```python
from build123d import *

# Parameters (mm, degrees)
BOSS_EXTRUDE1_DEPTH       = 15.875
SHELL1_T                  = -8.89
SKETCH2_R                 = 3.175
CUT_EXTRUDE1_DEPTH        = 7.35
F_4_40_TAPPED_HOLE1_D     = 2.2606
F_4_40_TAPPED_HOLE1_DEPTH = 7.62
F_4_40_TAPPED_HOLE1_TIP   = 0.679153


with BuildPart() as part:
    # Sketch1 → Boss-Extrude1 (new body, symmetric)
    with BuildSketch(Plane.XY):
        with BuildLine():
            ThreePointArc((0, -50.8), (-35.921024, -35.921024), (-50.8, 0))
            Line((-50.8, 0), (-67.31, 0))
            Line((-67.31, 0), (-67.31, -118.11))
            Line((-67.31, -118.11), (-88.9, -118.11))
            Line((-88.9, -118.11), (-88.9, -124.46))
            Line((-88.9, -124.46), (0, -124.46))
            Line((0, -124.46), (0, -50.8))
        make_face()
        with BuildLine():
            ThreePointArc((50.8, 0), (35.921024, -35.921024), (0, -50.8))
            Line((0, -50.8), (0, -124.46))
            Line((0, -124.46), (88.9, -124.46))
            Line((88.9, -124.46), (88.9, -118.11))
            Line((88.9, -118.11), (67.31, -118.11))
            Line((67.31, -118.11), (67.31, 0))
            Line((67.31, 0), (50.8, 0))
        make_face()
    extrude(amount=BOSS_EXTRUDE1_DEPTH, both=True)

    # Shell1
    shell1_openings = [part.faces().sort_by_distance(p)[0] for p in [
        (0, -77.216, 15.875),
        (0, -77.216, -15.875),
    ]]
    offset(amount=SHELL1_T, openings=shell1_openings)

    # Sketch2 → Cut-Extrude1 (cut, through all)
    with BuildSketch(Plane(origin=(0, -118.11, 0), x_dir=(1, 0, 0), z_dir=(0, 1, 0))):
        with Locations((-78.105, 0)):
            Circle(SKETCH2_R)
        with Locations((78.105, 0)):
            Circle(SKETCH2_R)
    extrude(amount=-CUT_EXTRUDE1_DEPTH, mode=Mode.SUBTRACT)

    # #4-40 Tapped Hole1
    with Locations(Plane(origin=(0, 0, 0), x_dir=(1, 0, 0), z_dir=(0, 1, 0))):
        with Locations((-57.658, 5.715), (-57.658, -6.985), (57.658, -6.985), (57.658, 5.715)):
            Hole(F_4_40_TAPPED_HOLE1_D / 2, depth=F_4_40_TAPPED_HOLE1_DEPTH)
            with Locations((0, 0, -(F_4_40_TAPPED_HOLE1_DEPTH + F_4_40_TAPPED_HOLE1_TIP / 2))):  # 118° drill point
                Cone(0, F_4_40_TAPPED_HOLE1_D / 2, F_4_40_TAPPED_HOLE1_TIP, mode=Mode.SUBTRACT)


solid = part.part
```
Read the model definition and answer for the solid it produces. Units are mm, in the model's axes. A direction names the side the tool comes from. Round coordinates to 2 decimals unless told otherwise and drop trailing zeros. Write each loop counter-clockwise with the first axis right and the second up, starting at its lowest first coordinate (ties: lowest second). Pieces come first, ordered by that corner, then holes. Notation, with made-up numbers: (48, 10) - (53, 10) arc R20 ccw to (53, 25) - close; hole circle Ø7 at (37, 4). An arc over 180 degrees is marked (long way). Use CSV: the item, a comma, the result in double quotes.
Q1. A tool of negligible diameter and unlimited length cuts with its end or side. For faces 4 (the flat face through (-58.42, -63, 0)), 5 (the flat face through (67.31, -60, 0)), 6 (the flat face through (-67.31, -58, 0)), from which of +Z, -Z, +X, -X, +Y, -Y can it reach the whole face along a straight path? Write none if from no direction.
Values:
face 4,"+Z, -Z"
face 5,"+Z, -Z, +X, +Y"
face 6,"+Z, -Z, -X, +Y"
Q2. Find section B-B, the plane y = -62.5. Write down the section's boundary in (x, z) (3 decimals), then the cut area to 3 significant figures.
Values:
outline,"(-67.31, -15.875) - (-58.42, -15.875) - (-58.42, 15.875) - (-67.31, 15.875) - close; (58.42, -15.875) - (67.31, -15.875) - (67.31, 15.875) - (58.42, 15.875) - close"
area,"565 mm²"
Q3. Determine the mould class of faces 1 (the cylindrical face through (-81.277, -121.241, -0.14)), 2 (the flat face through (58.42, -65, 0)), 3 (the flat face through (78, -118.11, 4)) for opening direction Y: +Y half, -Y half, draft (parallel to the pull), parting line (faces both ways), or undercut.
Values:
face 1,"draft"
face 2,"undercut"
face 3,"+Y half"
Q4. Straight lines are drawn through the part: line 1 along X through (y, z) = (-122, 0); line 2 along X through (y, z) = (-86.5, -12.5); line 3 along X through (y, z) = (-119, -2.5). For each, find the intervals that lie inside material, in ascending order.
Values:
line 1,"x = -88.9 to -81.28, -74.93 to 74.93, 81.28 to 88.9"
line 2,"x = -67.31 to -58.42, 58.42 to 67.31"
line 3,"x = -88.9 to -80.06, -76.15 to 76.15, 80.06 to 88.9"
Q5. Find section A-A, the plane z = 0. Write down the section's boundary in (x, y), then the cut area to 3 significant figures.
Values:
outline,"(-88.9, -124.46) - (-81.28, -124.46) - (-81.28, -118.11) - (-88.9, -118.11) - close; (-74.93, -124.46) - (74.93, -124.46) - (74.93, -118.11) - (67.31, -118.11) - (67.31, 0) - (50.8, 0) arc R50.8 cw to (0, -50.8) arc R50.8 cw to (-50.8, 0) - (-67.31, 0) - (-67.31, -118.11) - (-74.93, -118.11) - close; (81.28, -124.46) - (88.9, -124.46) - (88.9, -118.11) - (81.28, -118.11) - close; hole (-58.42, -115.57) - (58.42, -115.57) - (58.42, -12.25) arc R59.69 cw to (0, -59.69) arc R59.69 cw to (-58.42, -12.25) - close"
area,"4,970 mm²"
Q6. Each of these flat-tipped pins is pushed along its axis until it touches: pin 1 Ø8 at (x, z) = (-34, 5) entering from +Y; pin 2 Ø3.5 at (x, z) = (-57.658, -5.715) entering from +Y; pin 3 Ø3 at (y, z) = (-85, 9.5) entering from -X; pin 4 Ø16 at (x, z) = (16, -3.5) entering from +Y. Where does it stop, or does it pass through?
Values:
pin 1,"stops at y = -33.71"
pin 2,"stops at y = 0"
pin 3,"stops at x = -67.31"
pin 4,"stops at y = -44.77"
Q7. Find section D-D, the plane x = -28. Write down the section's boundary in (y, z) (3 decimals).
Values:
outline,"(-124.46, -15.875) - (-115.57, -15.875) - (-115.57, 15.875) - (-124.46, 15.875) - close; (-52.715, -15.875) - (-42.387, -15.875) - (-42.387, 15.875) - (-52.715, 15.875) - close"
Q8. Find section C-C, the plane z = -13.5. Write down the section's boundary in (x, y).
Values:
outline,"(-88.9, -124.46) - (88.9, -124.46) - (88.9, -118.11) - (67.31, -118.11) - (67.31, 0) - (50.8, 0) arc R50.8 cw to (0, -50.8) arc R50.8 cw to (-50.8, 0) - (-67.31, 0) - (-67.31, -118.11) - (-88.9, -118.11) - close; hole (-58.42, -115.57) - (58.42, -115.57) - (58.42, -12.25) arc R59.69 cw to (0, -59.69) arc R59.69 cw to (-58.42, -12.25) - close"
